Geometry check sheet. Reference: the model listing, model coordinates, mm. Give positions to 0.01 mm unless a question says otherwise; leave off trailing zeros. Loops run counter-clockwise (first coordinate to the right, second up) from the corner with the lowest first, then second, coordinate; pieces in that order, holes last. Notation, with made-up numbers: (65, 86.25) -> (77, 86.25) arc R12 ccw to (77, 106.25) -> close; hole circle Ø1 at (85.25, 25). An arc over 180 degrees is marked (long way). Answer as a JSON object with one key per item and string values.
from build123d import *

# Parameters (mm, degrees)
F0_W     = 1954
F0_H     = 494
F1_DEPTH = 3
F2_W     = 1954
F2_H     = 30
F3_DEPTH = 5
F4_W     = 1954
F4_H     = 6.620756
F5_DEPTH = 30


with BuildPart() as f1:
    # F0 (on Front) → F1 (new body)
    with BuildSketch(Plane.XZ):
        Rectangle(F0_W, F0_H)
    extrude(amount=F1_DEPTH)

    # F2 (on face) → F3 (join)
    with BuildSketch(Plane.XZ.offset(3)):
        with Locations((0, 232)):
            Rectangle(F2_W, F2_H)
        with Locations((0, -232)):
            Rectangle(F2_W, F2_H)
    extrude(amount=F3_DEPTH)

    # F4 (on face) → F5 (join)
    with BuildSketch(Plane.XZ.offset(8)):
        with Locations((0, 243.689622)):
            Rectangle(F4_W, F4_H)
        with Locations((0, -243.689622)):
            Rectangle(F4_W, F4_H)
    extrude(amount=F5_DEPTH)


solid = f1.part
1) Section check B-B on x = -452. Record the cut outline in (y, z).
Geometry check:
{"outline": "(-38, -247) -> (0, -247) -> (0, 247) -> (-38, 247) -> (-38, 240.38) -> (-8, 240.38) -> (-8, 217) -> (-3, 217) -> (-3, -217) -> (-8, -217) -> (-8, -240.38) -> (-38, -240.38) -> close"}
2) Material ranges on line 1 along Z through (x, y) = (-393.5, -26); line 2 along Z through (x, y) = (875.5, -4.5); line 3 along Y through (x, z) = (-171, 42.5), recorded low to high. Write a range as from..to.
Geometry check:
{"line 1": "z = -247..-240.38, 240.38..247", "line 2": "z = -247..-217, 217..247", "line 3": "y = -3..0"}
3) Depth check by flat-ended pin: P1, Ø1, axis at x = -111.5, z = -130.5, coming from the -Y side; P2, Ø6, axis at x = -368.5, z = -87.5, coming from the +Y side. Enter the tip coordinate at first touch or a pass-through.
Geometry check:
{"P1": "stops at y = -3", "P2": "stops at y = 0"}
4) Section check C-C on z = 193. Record the cut outline in (x, y).
Geometry check:
{"outline": "(-977, -3) -> (977, -3) -> (977, 0) -> (-977, 0) -> close"}
5) Draft check along Z on faces 1 (the face through (977, -2, -1)), 2 (the face through (-14, -3, 3)), 3 (the face through (-14, -19, 247)), 4 (the face through (-14, -19, -247)). Enter one of: pulls with the +Z half, pulls with the -Z half, needs draft (parallel to the pull), parting line crosses it, or undercut.
Geometry check:
{"face 1": "needs draft", "face 2": "undercut", "face 3": "pulls with the +Z half", "face 4": "pulls with the -Z half"}
6) Section check A-A on y = -26. Record the cut outline in (x, z), plus the area to 3 significant figures.
Geometry check:
{"outline": "(-977, -247) -> (977, -247) -> (977, -240.38) -> (-977, -240.38) -> close; (-977, 240.38) -> (977, 240.38) -> (977, 247) -> (-977, 247) -> close", "area": "25,900 mm2"}
